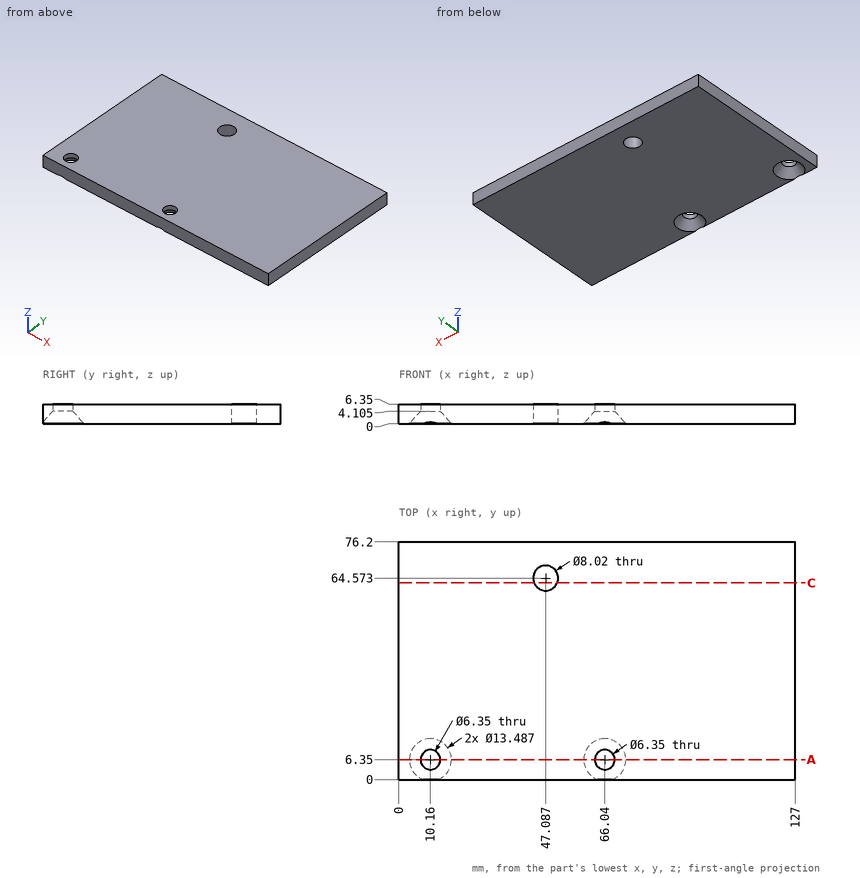
Answer from the drawing. Dimensions are ordinates in mm from the lowest x, y and z of the part. Round coordinates to 2 decimals unless told otherwise and drop trailing zeros. Write each loop counter-clockwise with the first axis right and the second up, starting at its lowest first coordinate (ties: lowest second). Pieces come first, ordered by that corner, then holes. Notation, with made-up numbers: (31.5, -0.5) - (50.5, -0.5) arc R25 cw to (50.5, 12.5) - close; hole circle Ø5 at (67.5, 68.5). An arc over 180 degrees is marked (long way). One line per item, written item: value.
Q1. Find section C-C (y = 63). Determine the outline of the cut face in (x, z).
The answers:
outline: (0, 0) - (43.4, 0) - (43.4, 6.35) - (0, 6.35) - close; (50.78, 0) - (127, 0) - (127, 6.35) - (50.78, 6.35) - close
Q2. This flat-tipped pin is pushed along its axis until it touches: P1, Ø7.5, axis at x = 10.16, y = 6.35, coming from the -Z side (1 decimal). Where does it stop, or does it pass through?
The answers:
P1: stops at z = 3.4
Q3. Straight lines are drawn through the part: line 1 (X direction, y = 6.35, z = 5.25) (1 decimal); line 2 (X direction, y = 8, z = 1.75) (1 decimal); line 3 (Y direction, x = 10.16, z = 4.8) (1 decimal). For each, find the intervals that lie inside material, in ascending order. Write a range as from..to.
The answers:
line 1: x = 0..7, 13.3..62.9, 69.2..127
line 2: x = 0..5.2, 15.1..61.1, 71..127
line 3: y = 0..3.2, 9.5..76.2
Q4. Find section A-A (y = 6.35). Count the separate pieces of the cut face and the enclosed holes in it.
The answers:
separate pieces: 3
enclosed holes: 0
